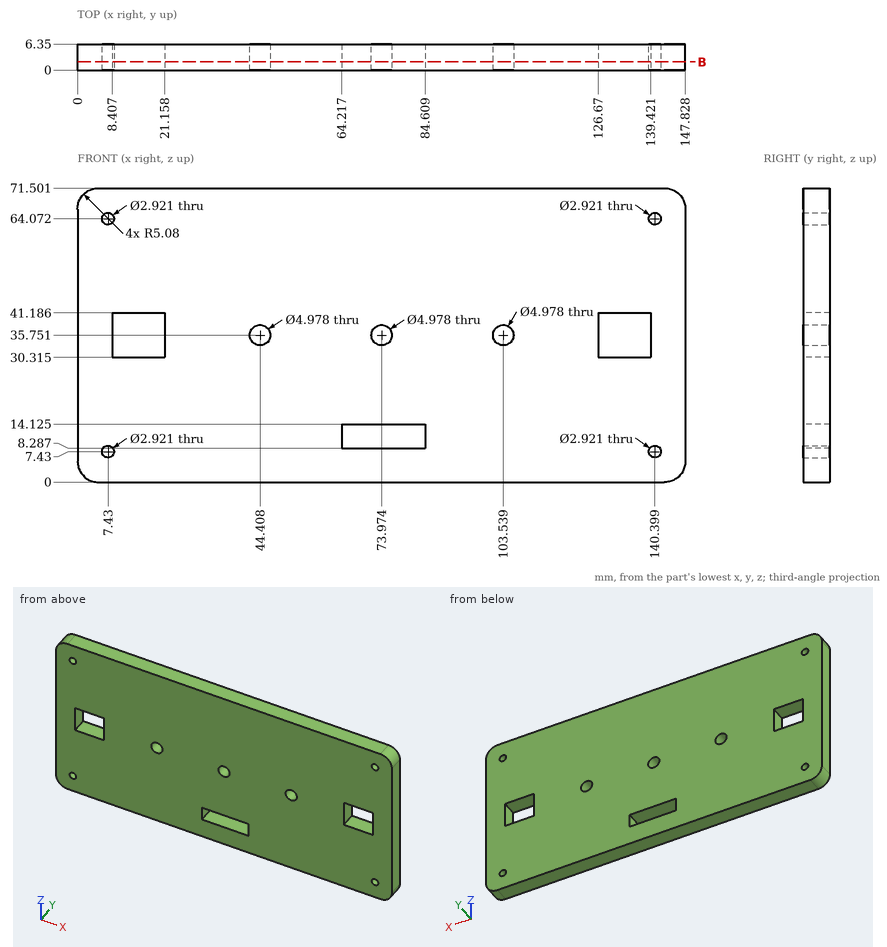
Geometry check sheet. Reference: drawing and pictorial views, mm from the part's lowest x, y, z. Round coordinates to 2 decimals unless told otherwise and drop trailing zeros. Write item = value, one per line. Start each with the question number.
Q1. Depth check by flat-ended pin: P1, Ø2.5, axis at x = 140.4, z = 64.07, coming from the +Y side. Enter the tip coordinate at first touch or a pass-through.
Q2. Section check B-B (y = 2). Count the separate pieces of the cut face and the enclosed holes in it, plus the area to 3 significant figures.
Q3. Thickness scan on L1, parallel to Z at x = 74, y = 4 (1 decimal); L2, parallel to X at y = 5.5, z = 34 (1 decimal); L3, parallel to Z at x = 79, y = 2.25 (1 decimal). Record the ranges inside material, lowest first.
Derived:
q1.P1 = through
q2.separate_pieces = 1
q2.enclosed_holes = 10
q2.area = 10,100 mm^2
q3.L1 = 0 to 8.3, 14.1 to 33.3, 38.2 to 71.5
q3.L2 = 0 to 8.4, 21.2 to 42.6, 46.2 to 72.2, 75.7 to 101.8, 105.3 to 126.7, 139.4 to 147.8
q3.L3 = 0 to 8.3, 14.1 to 71.5
